from build123d import *

# Parameters (mm, degrees)
BASE_FLANGE1_START       = -3.175
BASE_FLANGE1_DEPTH       = 3.175
EDGE_FLANGE1_START       = -0.3353435
EDGE_FLANGE1_DEPTH       = 0.3353435
EDGE_FLANGE1_START_2     = -3.175
EDGE_FLANGE1_2_DEPTH     = 3.175
EDGE_FLANGE1_START_3     = -44.45
EDGE_FLANGE1_3_OUTLINE_W = 136.033825791
EDGE_FLANGE1_3_OUTLINE_H = 3.175
EDGE_FLANGE1_3_DEPTH     = 38.1
EDGE_FLANGE1_START_4     = -139.7
EDGE_FLANGE1_4_DEPTH     = 136.033825791
EDGE_FLANGE1_START_5     = 3.666174209
EDGE_FLANGE1_5_DEPTH     = 136.033825791
EDGE_FLANGE1_6_DEPTH     = 146.096388787
EDGE_FLANGE1_START_6     = -69.85
EDGE_FLANGE1_7_DEPTH     = 209.55
FILLET2_R                = 220.82
SKETCH15_R               = 3.3734375
CUT_EXTRUDE1_DEPTH       = 206.261094571
SKETCH16_R               = 3.3734375
CUT_EXTRUDE2_DEPTH       = 206.261094571
FILLET3_R                = 3.175


with BuildPart() as part:
    # Base-Flange1: read off the stored shape, not the designer's step
    # Base-Flange1 outline → Base-Flange1 (new body)
    with BuildSketch(Plane.XY.offset(BASE_FLANGE1_START)):
        Polygon((69.85, 120.983748909), (31.595939562, 143.620651524), (-25.447777456, 44.572661394), (-139.747711611, 44.449974394), (-139.7, 0), (0, 0), align=None)
    extrude(amount=BASE_FLANGE1_DEPTH)

    # Edge-Flange1: read off the stored shape, not the designer's step
    # Edge-Flange1 outline → Edge-Flange1 (cut)
    with BuildSketch(Plane.XY.offset(EDGE_FLANGE1_START)):
        Polygon((-139.7, 7.9375), (-139.708519936, 7.9375), (-139.7, 0), (0, 0), (1.833087105, 3.175), (69.85, 120.983748909), (63.01852425, 125.026285819), (62.975923357, 124.952498909), (64.350738686, 124.158748909), (67.100369343, 122.571248909), (-0.916543552, 4.7625), (-3.666174209, 6.35), (-3.666174209, 3.175), (-139.7, 3.175), align=None)
    extrude(amount=EDGE_FLANGE1_DEPTH, mode=Mode.SUBTRACT)

    # Edge-Flange1 2 outline → Edge-Flange1 2 (cut)
    with BuildSketch(Plane.XY.offset(EDGE_FLANGE1_START_2)):
        Polygon((-139.7, 7.9375), (-139.708519936, 7.9375), (-139.7, 0), align=None)
        Polygon((-3.666174209, 6.35), (-3.666174209, 0), (0, 0), (1.833087105, 3.175), align=None)
        Polygon((64.350738686, 124.158748909), (69.85, 120.983748909), (63.01852425, 125.026285819), (62.975923357, 124.952498909), align=None)
    extrude(amount=EDGE_FLANGE1_2_DEPTH, mode=Mode.SUBTRACT)



with BuildPart() as body_2:
    # Edge-Flange1 3 outline → Edge-Flange1 3 (new body)
    with BuildSketch(Plane.XY.offset(EDGE_FLANGE1_START_3)):
        with Locations((-71.683087105, 1.5875)):
            Rectangle(EDGE_FLANGE1_3_OUTLINE_W, EDGE_FLANGE1_3_OUTLINE_H)
        Polygon((-0.916543552, 4.7625), (1.833087105, 3.175), (69.85, 120.983748909), (67.100369343, 122.571248909), align=None)
    extrude(amount=EDGE_FLANGE1_3_DEPTH)


with BuildPart() as part_1:
    add(part.part)

    add(body_2.part)  # Edge-Flange1 4 merges body 2
    # Edge-Flange1 4 outline → Edge-Flange1 4 (add)
    with BuildSketch(Plane.YZ.offset(EDGE_FLANGE1_START_4)):
        with BuildLine():
            ThreePointArc((0.850738685, -3.175), (0.216371003, -4.706499064), (0, -6.35))
            Line((0, -6.35), (3.175, -6.35))
            ThreePointArc((3.175, -6.35), (4.10493597, -4.10493597), (6.35, -3.175))
            Line((6.35, -3.175), (0.850738685, -3.175))
        make_face()
    extrude(amount=EDGE_FLANGE1_4_DEPTH)

    # Edge-Flange1 5 outline → Edge-Flange1 5 (add)
    with BuildSketch(Plane(origin=(0, 0, 0), x_dir=(0.866025403784418, -0.500000000000036, 0), z_dir=(0.500000000000036, 0.866025403784418, 0)).offset(EDGE_FLANGE1_START_5)):
        with BuildLine():
            ThreePointArc((-0.850738685, 3.175), (-0.216371003, 4.706499064), (0, 6.35))
            Line((0, 6.35), (-3.175, 6.35))
            ThreePointArc((-3.175, 6.35), (-4.10493597, 4.10493597), (-6.35, 3.175))
            Line((-6.35, 3.175), (-0.850738685, 3.175))
        make_face()
    extrude(amount=EDGE_FLANGE1_5_DEPTH)

    # Edge-Flange1 6 outline → Edge-Flange1 6 (cut)
    with BuildSketch(Plane.YZ.offset(EDGE_FLANGE1_START_4)):
        with BuildLine():
            Line((0, -3.175), (0.850738685, -3.175))
            ThreePointArc((0.850738685, -3.175), (3.174999999, -0.850738686), (6.35, 0))
            Line((6.35, 0), (3.175, 0))
            Line((3.175, 0), (3.175, -0.3353435))
            Line((3.175, -0.3353435), (0, -0.3353435))
            Line((0, -0.3353435), (0, -3.175))
        make_face()
    extrude(amount=EDGE_FLANGE1_6_DEPTH, mode=Mode.SUBTRACT)

    # Edge-Flange1 7 outline → Edge-Flange1 7 (cut)
    with BuildSketch(Plane(origin=(0, 0, 0), x_dir=(0.866025403784418, -0.500000000000036, 0), z_dir=(0.500000000000036, 0.866025403784418, 0)).offset(EDGE_FLANGE1_START_6)):
        with BuildLine():
            Line((0, 3.175), (-0.850738685, 3.175))
            ThreePointArc((-0.850738685, 3.175), (-3.174999999, 0.850738686), (-6.35, 0))
            Line((-6.35, 0), (-3.175, 0))
            Line((-3.175, 0), (-3.175, 0.3353435))
            Line((-3.175, 0.3353435), (0, 0.3353435))
            Line((0, 0.3353435), (0, 3.175))
        make_face()
    extrude(amount=EDGE_FLANGE1_7_DEPTH, mode=Mode.SUBTRACT)

    # Fillet2
    # the kernel refuses this fillet: 220.82 mm, written as the material it adds along each edge
    with BuildSketch(Plane(origin=(-25.447777456, 44.572661394, -3.175), x_dir=(0.49907014013952505, 0.8665615934376014, 0), z_dir=(0, 0, 1))) as fillet2_piece_1:
        with BuildLine():
            CenterArc((127.27037084, 220.438748591), FILLET2_R, 213.36733761, 53.265324779)
            Line((-57.149999999, 98.986703653), (0, 0))
            Line((0, 0), (114.3, 0))
        make_face()
    extrude(amount=3.175)

    # Sketch15 → Cut-Extrude1 (cut, through all)
    with BuildSketch(Plane(origin=(0, 0, 0), x_dir=(0, 0, -1), z_dir=(0.8660254037844249, -0.5000000000000239, 3.506248131957107e-15))):
        with Locations(Location((25.4, 104.22382, 0), (0, 0, 90))):
            Circle(SKETCH15_R)
        with Locations(Location((25.4, 46.284161604, 0), (0, 0, 90))):
            Circle(SKETCH15_R)
    extrude(amount=-CUT_EXTRUDE1_DEPTH, mode=Mode.SUBTRACT)

    # Sketch16 → Cut-Extrude2 (cut, through all)
    with BuildSketch(Plane.XZ):
        with Locations(Location((-104.22382, -25.4, 0), (0, 0, 270))):
            Circle(SKETCH16_R)
        with Locations(Location((-46.284161686, -25.4, 0), (0, 0, 270))):
            Circle(SKETCH16_R)
    extrude(amount=-CUT_EXTRUDE2_DEPTH, mode=Mode.SUBTRACT)

    # Fillet3
    fillet3_edges = [part_1.edges().sort_by_distance(p)[0] for p in [
        (31.595939562, 143.620651524, -1.5875),
        (-139.747711611, 44.449974394, -1.5875),
        (-3.666174209, 1.5875, -44.45),
        (-139.7, 1.5875, -44.45),
        (68.475184671, 121.777498909, -44.45),
        (0.458271776, 3.96875, -44.45),
    ]]
    fillet(fillet3_edges, radius=FILLET3_R)


solid = part_1.part
Part model, mm, in its own coordinate system. A direction names the side the tool comes from. Coordinates: 2 decimals unless noted, no trailing zeros. Loops run counter-clockwise (first coordinate to the right, second up) from the corner with the lowest first, then second, coordinate; pieces in that order, holes last. Notation, with made-up numbers: (81, -25.75) - (89, -25.75) arc R23 cw to (89, 5.25) - close; hole circle Ø11 at (-33.5, -30.75). An arc over 180 degrees is marked (long way). Write each question's results on one line, items separated by ' | '. Start each with the question number.
Q1. Slice it at B-B on z = -25.4. Give the number of separate pieces and of enclosed holes in the cut face, and give its area (3 significant figures).
Q2. Slice it at C-C on x = -63. Give the cut face in (y, z) (3 decimals), and give its area (3 significant figures).
Q3. Slice it at D-D on y = 128. Give the cut face in (x, z) (3 decimals).
Q4. Two-plate mould, pull along X, no slides. Class faces 3 (the cylindrical face through (-45.271, 1.565, -28.618)), 4 (the cylindrical face through (68, 121, -43.5)), 5 (the flat face through (-139.7, 2, -20)): +X half, -X half, draft (parallel to the pull), parting line (faces both ways), or undercut.
Q5. Which spindle directions (+Z, -Z, +X, -X, +Y, -Y) get a long thin tool onto all of the face, cutting with end or side? Do faces 1 (the cylindrical face through (20.543, 38.713, -23.12)), 2 (the flat face through (-32, 64, -3.175)). Say none if no direction does.
Q6. Drop flat-ended pins along their axis: pin 1 Ø2.5 at (y, z) = (5, -19.5) entering from -X; pin 2 Ø19 at (x, z) = (-74, -18) entering from +Y (3 decimals); pin 3 Ø1 at (y, z) = (122, -32.5) entering from -X; pin 4 Ø4 at (x, z) = (-46.28, -25.4) entering from +Y (1 decimal). Give the stop position or say it passes through.
Q7. Probe line 1 along X through (y, z) = (1, -25); line 2 along Y through (x, z) = (-78.5, -34) (3 decimals); line 3 along Z through (x, y) = (4.5, 36) (3 decimals). List the from-to ranges inside material, lowest first.
Answer:
1) separate pieces: 6 | enclosed holes: 0 | area: 778 mm2
2) outline: (0, -44.45) - (3.175, -44.45) - (3.175, -6.35) arc R3.175 cw to (6.35, -3.175) - (63.208, -3.175) - (63.208, 0) - (6.35, 0) arc R6.35 ccw to (0, -6.35) - close | area: 325 mm2
3) outline: (20.328, -3.175) - (57.993, -3.175) - (57.993, 0) - (20.328, 0) - close
4) face 3: undercut | face 4: +X half | face 5: -X half
5) face 1: none | face 2: -Z, -X, +Y
6) pin 1: stops at x = -0.92 | pin 2: stops at y = 3.175 | pin 3: stops at x = 66.48 | pin 4: passes through
7) line 1: x = -139.7 to -107.57, -100.87 to -49.63, -42.93 to -3.67 | line 2: y = 0 to 3.175 | line 3: z = -3.175 to 0
